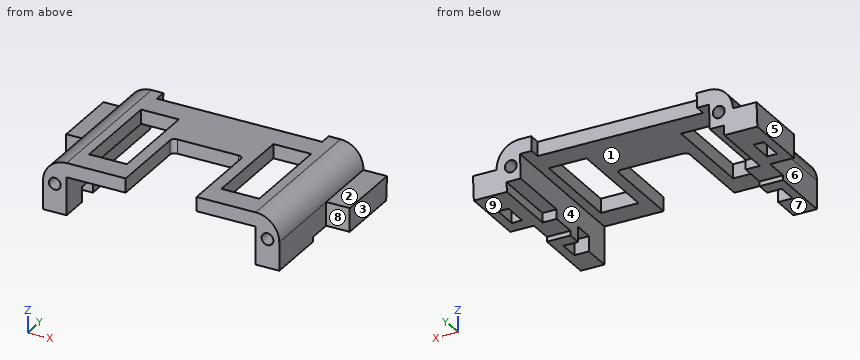
from build123d import *

# Parameters (mm, degrees)
BOSS_EXTRUDE1_DEPTH = 16.32
SKETCH3_W           = 8
SKETCH3_H           = 20
SKETCH3_W_2         = 15
SKETCH3_H_2         = 18
CUT_EXTRUDE1_DEPTH  = 4
SKETCH4_W           = 1
SKETCH4_H           = 19.64
CUT_EXTRUDE2_DEPTH  = 27.5
FILLET1_R           = 5
CUT_EXTRUDE3_DEPTH  = 26
BOSS_EXTRUDE2_START = -25
BOSS_EXTRUDE2_DEPTH = 5
BOSS_EXTRUDE3_START = 25
BOSS_EXTRUDE3_DEPTH = 5
SKETCH7_R           = 1.25
CUT_EXTRUDE4_DEPTH  = 5
SKETCH8_W           = 35
SKETCH8_H           = 5
CUT_EXTRUDE5_DEPTH  = 5
CUT_EXTRUDE6_START  = -10
SKETCH9_W           = 2.2
SKETCH9_H           = 5.2
CUT_EXTRUDE6_DEPTH  = 3.2
CUT_EXTRUDE7_START  = -16.32
SKETCH10_R          = 1.25
CUT_EXTRUDE7_DEPTH  = 5
CUT_EXTRUDE8_START  = -11
SKETCH11_W          = 3.2
SKETCH11_H          = 4.2
CUT_EXTRUDE8_DEPTH  = 3.2
CUT_EXTRUDE9_START  = 2
SKETCH12_W          = 3
SKETCH12_H          = 2
CUT_EXTRUDE9_DEPTH  = 15
FILLET3_R           = 1


with BuildPart() as part:
    # Sketch2 → Boss-Extrude1 (new body, symmetric)
    with BuildSketch(Plane(origin=(0, 0, 0), x_dir=(1, 0, 0), z_dir=(0, 1, 0))):
        Polygon((-25, 0), (25, 0), (25, 11), (20, 11), (20, 3), (-20, 3), (-20, 11), (-25, 11), align=None)
    extrude(amount=BOSS_EXTRUDE1_DEPTH, both=True)

    # Sketch3 → Cut-Extrude1 (cut)
    with BuildSketch(Plane.XY):
        with Locations((14, -1.32)):
            Rectangle(SKETCH3_W, SKETCH3_H)
        with Locations((-14, -1.32)):
            Rectangle(SKETCH3_W, SKETCH3_H)
        with Locations((0, -7.32)):
            Rectangle(SKETCH3_W_2, SKETCH3_H_2)
    extrude(amount=-CUT_EXTRUDE1_DEPTH, mode=Mode.SUBTRACT)

    # Sketch4 → Cut-Extrude2 (cut, symmetric)
    with BuildSketch(Plane(origin=(0, 0, 0), x_dir=(0, 0, -1), z_dir=(1, 0, 0))):
        with Locations((10.5, 6.5)):
            Rectangle(SKETCH4_W, SKETCH4_H)
    extrude(amount=CUT_EXTRUDE2_DEPTH, both=True, mode=Mode.SUBTRACT)

    # Fillet1
    fillet1_edges = [part.edges().sort_by_distance(p)[0] for p in [
        (25, 0, 0),
        (-25, 0, 0),
    ]]
    fillet(fillet1_edges, radius=FILLET1_R)

    # Sketch5 → Cut-Extrude3 (cut, symmetric)
    with BuildSketch(Plane(origin=(0, 0, 0), x_dir=(0, 0, -1), z_dir=(1, 0, 0))):
        Polygon((10, 16.32), (0, 16.32), (10, 15.68), align=None)
    extrude(amount=CUT_EXTRUDE3_DEPTH, both=True, mode=Mode.SUBTRACT)

    # Sketch6 → Boss-Extrude2 (add)
    with BuildSketch(Plane(origin=(0, 0, 0), x_dir=(0, 0, -1), z_dir=(1, 0, 0)).offset(BOSS_EXTRUDE2_START)):
        Polygon((10, 15.68), (5, 16), (5, 1.68), (10, 1.68), align=None)
    extrude(amount=-BOSS_EXTRUDE2_DEPTH)

    # Sketch6<2> → Boss-Extrude3 (add)
    with BuildSketch(Plane(origin=(0, 0, 0), x_dir=(0, 0, -1), z_dir=(1, 0, 0)).offset(BOSS_EXTRUDE3_START)):
        Polygon((10, 15.68), (5, 16), (5, 1.68), (10, 1.68), align=None)
    extrude(amount=BOSS_EXTRUDE3_DEPTH)

    # Sketch7 → Cut-Extrude4 (cut)
    with BuildSketch(Plane(origin=(0, 16.253425967, -1.040219262), x_dir=(1, 0, 0), z_dir=(0, 0.99795827, -0.063869329))):
        with Locations((22, 3.978111617)):
            Circle(SKETCH7_R)
        with Locations((-22, 3.978111617)):
            Circle(SKETCH7_R)
    extrude(amount=-CUT_EXTRUDE4_DEPTH, mode=Mode.SUBTRACT)

    # Sketch8 → Cut-Extrude5 (cut)
    with BuildSketch(Plane.XY):
        with Locations((0, 16.32)):
            Rectangle(SKETCH8_W, SKETCH8_H)
    extrude(amount=-CUT_EXTRUDE5_DEPTH, mode=Mode.SUBTRACT)

    # Sketch9 → Cut-Extrude6 (cut)
    with BuildSketch(Plane.XY.offset(CUT_EXTRUDE6_START)):
        with Locations((-27, 7.18)):
            Rectangle(SKETCH9_W, SKETCH9_H)
        with Locations((27, 7.18)):
            Rectangle(SKETCH9_W, SKETCH9_H)
    extrude(amount=CUT_EXTRUDE6_DEPTH, mode=Mode.SUBTRACT)

    # Sketch10 → Cut-Extrude7 (cut)
    with BuildSketch(Plane(origin=(0, 0, 0), x_dir=(1, 0, 0), z_dir=(0, 1, 0)).offset(CUT_EXTRUDE7_START)):
        with Locations((-22.5, 5)):
            Circle(SKETCH10_R)
        with Locations((22.5, 5)):
            Circle(SKETCH10_R)
    extrude(amount=CUT_EXTRUDE7_DEPTH, mode=Mode.SUBTRACT)

    # Sketch11 → Cut-Extrude8 (cut)
    with BuildSketch(Plane.XY.offset(CUT_EXTRUDE8_START)):
        with Locations((21.5, -8.32)):
            Rectangle(SKETCH11_W, SKETCH11_H)
        with Locations((-21.5, -8.32)):
            Rectangle(SKETCH11_W, SKETCH11_H)
    extrude(amount=CUT_EXTRUDE8_DEPTH, mode=Mode.SUBTRACT)

    # Sketch12 → Cut-Extrude9 (cut)
    with BuildSketch(Plane(origin=(0, 0, 0), x_dir=(1, 0, 0), z_dir=(0, 1, 0)).offset(CUT_EXTRUDE9_START)):
        with Locations((21.5, 9)):
            Rectangle(SKETCH12_W, SKETCH12_H)
        with Locations((-21.5, 9)):
            Rectangle(SKETCH12_W, SKETCH12_H)
    extrude(amount=CUT_EXTRUDE9_DEPTH, mode=Mode.SUBTRACT)

    # Fillet3
    fillet3_edges = [part.edges().sort_by_distance(p)[0] for p in [
        (-7.5, 1.68, -1.5),
        (7.5, 1.68, -1.5),
    ]]
    fillet(fillet3_edges, radius=FILLET3_R)


solid = part.part
Design review of the part built by this model. Coordinates are the model's own, in mm. Face numbers are marked on the shaded views. A direction names the side the tool comes from. Give positions to 0.01 mm unless a question says otherwise; leave off trailing zeros. Write each loop counter-clockwise with the first axis right and the second up, starting at its lowest first coordinate (ties: lowest second). Pieces come first, ordered by that corner, then holes. Notation, with made-up numbers: M 41.25,-21 L 63.25,-21 A32 cw 63.25,14 Z; hole C -19.75,20.25 d6. An arc over 180 degrees is marked long. Answer as a JSON object with one key per item and string values. Group by question number.
1) For line 1 along X through (y, z) = (-14.15, -5); line 2 along X through (y, z) = (-9, -8); line 3 along X through (y, z) = (-12, -7.75), list the stretches that pass through material, from the lowest coordinate up.
2) We need section B-B (x = 12.5). Give the boundary of the cut face in (y, z), and give its area (3 significant figures).
3) Clearance check with flat-ended pins moving along their axes: pin 1 Ø1.5 at (x, z) = (-2.5, -4.5) entering from -Y; pin 2 Ø5 at (x, z) = (-1, -2) entering from -Y; pin 3 Ø1.2 at (x, z) = (-22, -4.5) entering from -Y; pin 4 Ø1.5 at (x, y) = (-23.5, 8) entering from -Z. State where each tip first meets the part, or that it passes through.
4) We need section D-D (y = -8.5). Give the boundary of the cut face in (x, z).
5) We need section A-A (y = 7.5). Count the separate pieces of the cut face and the enclosed holes in it, and give its area (3 significant figures).
6) Mouldability with a two-part tool opening along X and no side actions: class the marked faces 1, 2, 3 and 4 as released by +X, released by -X, zero draft, split by the parting line, or undercut.
7) Tool access review of the marked faces 5, 6, 7, 8 and 9: name each direction out of +Z, -Z, +X, -X, +Y, -Y from which nothing blocks a thin tool from reaching the whole face with its end or side.
8) We need section C-C (y = -4). Give the boundary of the cut face in (x, z).
Answer key:
{
 "1": {"line 1": "x = -25 to -23.75, -21.25 to -20, 20 to 21.25, 23.75 to 25", "line 2": "x = -25 to -23.1, 23.1 to 25", "line 3": "x = -25 to -20, 20 to 25"},
 "2": {"outline": "M -16.32,-3 L -11.32,-3 L -11.32,0 L -16.32,0 Z; M 8.68,-3 L 13.82,-3 L 13.82,0 L 8.68,0 Z", "area": "30.4 mm²"},
 "3": {"pin 1": "passes through", "pin 2": "stops at y = 1.68", "pin 3": "stops at y = -16.32", "pin 4": "stops at z = -10"},
 "4": {"outline": "M -25,-11 L -23.1,-11 L -23.1,-7.8 L -20,-7.8 L -20,-3 L -18,-3 L -18,0 L -20,0 A5 ccw -25,-5 Z; M -10,-3 L -7.5,-3 L -7.5,0 L -10,0 Z; M 7.5,-3 L 10,-3 L 10,0 L 7.5,0 Z; M 18,-3 L 20,-3 L 20,-7.8 L 23.1,-7.8 L 23.1,-11 L 25,-11 L 25,-5 A5 ccw 20,0 L 18,0 Z"},
 "5": {"separate pieces": "3", "enclosed holes": "0", "area": "185 mm²"},
 "6": {"face 1": "undercut", "face 2": "zero draft", "face 3": "released by +X", "face 4": "undercut"},
 "7": {"face 5": "+Z, -Z, -X, +Y, -Y", "face 6": "+Z, -Z, -X, -Y", "face 7": "-Z, +X, -X, +Y, -Y", "face 8": "+Z, -Z, +X, -Y", "face 9": "-Z, +X, -X, +Y"},
 "8": {"outline": "M -25,-11 L -20,-11 L -20,-3 L -18,-3 L -18,0 L -20,0 A5 ccw -25,-5 Z; M -10,-3 L -7.5,-3 L -7.5,0 L -10,0 Z; M 7.5,-3 L 10,-3 L 10,0 L 7.5,0 Z; M 18,-3 L 20,-3 L 20,-11 L 25,-11 L 25,-5 A5 ccw 20,0 L 18,0 Z"}
}
